Work out the finished part from the listing and answer in its coordinate system (mm). Face numbers are marked on the shaded views. A direction names the side the tool comes from. Give positions to 0.01 mm unless a question says otherwise; leave off trailing zeros. Loops run counter-clockwise (first coordinate to the right, second up) from the corner with the lowest first, then second, coordinate; pieces in that order, holes last. Notation, with made-up numbers: (46, 69) - (96, 69) arc R29 cw to (96, 90) - close; hole circle Ø9 at (86, 50.5). An arc over 180 degrees is marked (long way). Use CSV: the item, a comma, the result in double quotes.
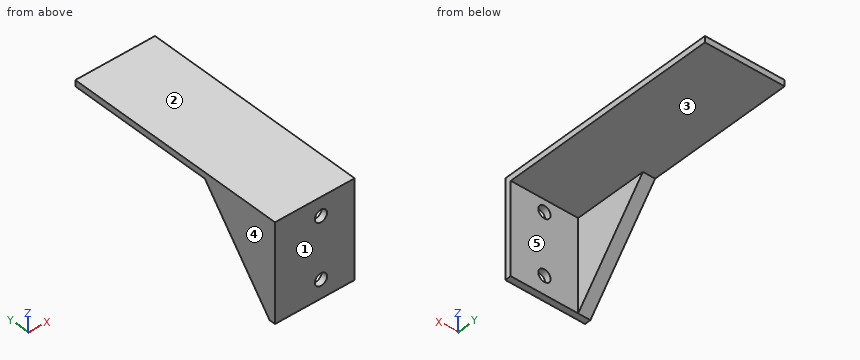
from build123d import *

# Parameters (mm, degrees)
BOSS_EXTRUDE1_DEPTH = 146.05
SKETCH2_W           = 63.5
SKETCH2_H           = 234.95
CUT_EXTRUDE1_DEPTH  = 146.05
BOSS_EXTRUDE2_DEPTH = 12.7
SKETCH4_R           = 6.35
CUT_EXTRUDE2_DEPTH  = 12.7


with BuildPart() as part:
    # Sketch1 → Boss-Extrude1 (new body)
    with BuildSketch(Plane(origin=(0, 0, 0), x_dir=(0, 0, -1), z_dir=(1, 0, 0))):
        Polygon((0, 0), (-101.6, 0), (-101.6, 6.35), (-101.6, 234.95), (-95.25, 234.95), (-95.25, 6.35), (0, 6.35), align=None)
    extrude(amount=BOSS_EXTRUDE1_DEPTH)

    # Sketch2 → Cut-Extrude1 (cut)
    with BuildSketch(Plane.XY.offset(101.6)):
        with Locations((31.75, 117.475)):
            Rectangle(SKETCH2_W, SKETCH2_H)
    extrude(amount=-CUT_EXTRUDE1_DEPTH, mode=Mode.SUBTRACT)

    # Sketch3 → Boss-Extrude2 (add)
    with BuildSketch(Plane.ZY.offset(-63.5)):
        Polygon((0, 6.35), (95.25, 82.55), (95.25, 6.35), align=None)
    extrude(amount=-BOSS_EXTRUDE2_DEPTH)

    # Sketch4 → Cut-Extrude2 (cut)
    with BuildSketch(Plane(origin=(0, 6.35, 0), x_dir=(1, 0, 0), z_dir=(0, 1, 0))):
        with Locations((111.125, -19.05)):
            Circle(SKETCH4_R)
        with Locations((111.125, -82.55)):
            Circle(SKETCH4_R)
    extrude(amount=-CUT_EXTRUDE2_DEPTH, mode=Mode.SUBTRACT)


solid = part.part
Item 1: A cutting plane is placed at D-D on z = 82.55. Determine the outline of the cut face in (x, y) (3 decimals).
Determined:
outline,"(63.5, 0) - (104.775, 0) - (104.775, 6.35) - (76.2, 6.35) - (76.2, 72.39) - (63.5, 72.39) - close; (117.475, 0) - (146.05, 0) - (146.05, 6.35) - (117.475, 6.35) - close"
Item 2: Find the intervals of material crossed by line 1 (X direction, y = 1, z = 19); line 2 (Z direction, x = 90, y = 170); line 3 (Y direction, x = 103.5, z = 41.5), in increasing order.
Determined:
line 1,"x = 63.5 to 104.78, 117.47 to 146.05"
line 2,"z = 95.25 to 101.6"
line 3,"y = 0 to 6.35"
Item 3: A cutting plane is placed at B-B on z = 68.5. Determine the outline of the cut face in (x, y), and give its area (3 significant figures).
Determined:
outline,"(63.5, 0) - (146.05, 0) - (146.05, 6.35) - (76.2, 6.35) - (76.2, 61.15) - (63.5, 61.15) - close"
area,"1,220 mm²"
Item 4: A cutting plane is placed at A-A on z = 19.05. Determine the outline of the cut face in (x, y) (3 decimals), and give its area (3 significant figures).
Determined:
outline,"(63.5, 0) - (104.775, 0) - (104.775, 6.35) - (76.2, 6.35) - (76.2, 21.59) - (63.5, 21.59) - close; (117.475, 0) - (146.05, 0) - (146.05, 6.35) - (117.475, 6.35) - close"
area,"637 mm²"
Item 5: Given P1, Ø4, axis at x = 116.5, y = 108.5, coming from the -Z side; P2, Ø7.5, axis at x = 111.125, z = 82.55, coming from the -Y side; P3, Ø10, axis at x = 118.5, z = 88, coming from the -Y side; P4, Ø12, axis at x = 119, z = 81, coming from the +Y side, each flat-ended and moving along its own axis, determine where each tip first touches the part or whether it passes through.
Determined:
P1,"stops at z = 95.25"
P2,"passes through"
P3,"stops at y = 0"
P4,"stops at y = 6.35"
Item 6: For the marked faces 4 and 5, determine the directions among +Z, -Z, +X, -X, +Y, -Y from which every point of the face is accessible in a straight line to the end or side of a thin tool.
Determined:
face 4,"+Z, -Z, -X, +Y, -Y"
face 5,"-Z, +X, +Y"
Item 7: The mould has two halves that part along Z. Classify the marked faces 1, 2 and 3: pulls with the +Z half, pulls with the -Z half, needs draft (parallel to the pull), parting line crosses it, or undercut.
Determined:
face 1,"needs draft"
face 2,"pulls with the +Z half"
face 3,"pulls with the -Z half"
Item 8: A cutting plane is placed at C-C on x = 129.5. Determine the outline of the cut face in (y, z).
Determined:
outline,"(0, 0) - (6.35, 0) - (6.35, 95.25) - (234.95, 95.25) - (234.95, 101.6) - (0, 101.6) - close"
